Build history of the part. All positions in model axes, mm. A direction names the side the tool comes from. Give positions to 0.01 mm unless a question says otherwise; leave off trailing zeros. Loops run counter-clockwise (first coordinate to the right, second up) from the corner with the lowest first, then second, coordinate; pieces in that order, holes last.
1) Band-saw the part on C-C on z = -2.5. State how many separate pieces and enclosed holes the cut face has, then the cut area to 3 significant figures.
2) 3-axis set-ups, long thin cutter, end or side, ignore diameter. For faces 4 (the flat face through (5.92, 42.93, 10.44)), 5 (the flat face through (-12, 103, 0)), 6 (the flat face through (-6.084, 42.93, 10.344)), 7 (the flat face through (2, 48, 8)), 8 (the conical face through (0.03, 38.26, 12.45)): which of +Z, -Z, +X, -X, +Y, -Y reach the whole face in a straight line?
3) Band-saw the part on B-B on y = 51. List the corners of the cut face in (x, z), then the cut area to 3 significant figures.
4) Band-saw the part on A-A on x = 41.75. List the corners of the cut face in (y, z), then the cut area to 3 significant figures.
5) Flat gauge pins, fed straight in: P1, Ø6, axis at x = -0.5, y = 117.5, coming from the +Z side; P2, Ø3, axis at y = 44, z = 0.5, coming from the +X side; P3, Ø11, axis at y = 45, z = 2.5, coming from the -X side. Where does each tip first touch, or does it go through?
6) Two-plate mould, pull along Y, no slides. Class faces 1 (the conical face through (0.03, 47.744, 12.443)), 2 (the conical face through (-10.8, 109.74, -6.2)), 3 (the flat face through (5.92, 103.41, 10.44)): +Y half, -Y half, draft (parallel to the pull), parting line (faces both ways), or undercut.
7) Wall check: line 1 (Y direction, x = -31.5, z = 19); line 2 (X direction, y = 44, z = 2); line 3 (Z direction, x = 41, y = 7). Give the ranges that are in metal, low to high.
```python
from build123d import *

# Parameters (mm, degrees)
EXTRUDE_1_DEPTH     = 10
EXTRUDE_2_DEPTH     = 13
SKETCH_5_R          = 5.25
CUT_EXTRUDE_1_DEPTH = 11


with BuildPart() as part:
    # Эскиз1 → Повернуть1 (revolve)
    with BuildSketch(Plane.XY, mode=Mode.PRIVATE) as revolve_1_sk:
        Polygon((0, 0), (-50, 0), (-50, 10), (-30, 10), (-22, 29), (-12, 29), (-12, 31), (-8, 35), (-8, 38), (-8, 48), (-8, 146), (-6, 148), (0, 148), align=None)
    revolve(revolve_1_sk.sketch.rotate(Axis((0, 0, 0), (0, 1, 0)), 180), axis=Axis((0, 0, 0), (0, 1, 0)))  # turned: the seam where the file's is

    # Эскиз2 → Бобышка-Вытянуть1 (add)
    with BuildSketch(Plane(origin=(0, 38, 0), x_dir=(1, 0, 0), z_dir=(0, 1, 0))):
        Polygon((0, 13.856406461), (-12, 6.92820323), (-12, -6.92820323), (0, -13.856406461), (12, -6.92820323), (12, 6.92820323), align=None)
    extrude(amount=EXTRUDE_1_DEPTH)

    # Эскиз3 → Бобышка-Вытянуть2 (add)
    with BuildSketch(Plane(origin=(0, 97, 0), x_dir=(1, 0, 0), z_dir=(0, 1, 0))):
        Polygon((12, 6.92820323), (0, 13.856406461), (-12, 6.92820323), (-12, -6.92820323), (0, -13.856406461), (12, -6.92820323), align=None)
    extrude(amount=EXTRUDE_2_DEPTH)

    # Эскиз4 → Вырез-Повернуть2 (revolve, cut)
    with BuildSketch(Plane.XY, mode=Mode.PRIVATE) as cut_revolve_2_sk:
        Polygon((-23.258330249, 110), (-12, 110), (-23.258330249, 103.5), align=None)
        Polygon((-23.258330249, 97), (-23.258330249, 103.5), (-12, 97), align=None)
        Polygon((-20.660254038, 48), (-20.660254038, 43), (-12, 48), align=None)
        Polygon((-20.660254038, 43), (-20.660254038, 38), (-12, 38), align=None)
    revolve(cut_revolve_2_sk.sketch.rotate(Axis((0, 148, 0), (0, -1, 0)), 180), axis=Axis((0, 148, 0), (0, -1, 0)), mode=Mode.SUBTRACT)  # turned: the seam where the file's is

    # Эскиз5 → Вырез-Вытянуть1 (cut, through all)
    with BuildSketch(Plane(origin=(0, 10, 0), x_dir=(1, 0, 0), z_dir=(0, 1, 0))):
        with Locations(Location((-41.75, 0, 0), (0, 0, 180))):  # turned: the seam where the file's is
            Circle(SKETCH_5_R)
        with Locations(Location((41.75, 0, 0), (0, 0, 180))):  # turned: the seam where the file's is
            Circle(SKETCH_5_R)
    extrude(amount=-CUT_EXTRUDE_1_DEPTH, mode=Mode.SUBTRACT)


solid = part.part
```
Findings below:
1. separate pieces: 3
1. enclosed holes: 0
1. area: 3,840 mm2
2. face 4: +Z, +X, +Y
2. face 5: +Z, -Z, -X, +Y
2. face 6: +Z, -X, +Y
2. face 7: none
2. face 8: +Z
3. outline: circle Ø16 at (0, 0)
3. area: 201 mm2
4. outline: (0, -27.51) - (10, -27.51) - (10, -5.25) - (0, -5.25) - close; (0, 5.25) - (10, 5.25) - (10, 27.51) - (0, 27.51) - close
4. area: 445 mm2
5. P1: stops at z = 8
5. P2: stops at x = 12
5. P3: stops at x = -12
6. face 1: undercut
6. face 2: +Y half
6. face 3: draft
7. line 1: y = 0 to 10
7. line 2: x = -12 to 12
7. line 3: z = -28.62 to -5.2, 5.2 to 28.62
